```python
from build123d import *

# Parameters (mm, degrees)
F0_W     = 93.756211
F0_H     = 57.899028
F1_DEPTH = 25.4
F2_W     = 93.756211
F2_H     = 57.899028
F3_DEPTH = 7.105513
F6_DEPTH = 25.4


with BuildPart() as f1:
    # F0 (on Top) → F1 (new body)
    with BuildSketch(Plane.XY):
        with Locations((11.77345, 3.361836)):
            Rectangle(F0_W, F0_H)
        with BuildLine():
            Line((39.601556, -12.887678), (-16.054655, -12.887678))
            ThreePointArc((-16.054655, -12.887678), (-20.544783, -11.027806), (-22.404655, -6.537678))
            Line((-22.404655, -6.537678), (-22.404655, 13.26135))
            ThreePointArc((-22.404655, 13.26135), (-20.544783, 17.751478), (-16.054655, 19.61135))
            Line((-16.054655, 19.61135), (39.601556, 19.61135))
            ThreePointArc((39.601556, 19.61135), (44.091684, 17.751478), (45.951556, 13.26135))
            Line((45.951556, 13.26135), (45.951556, -6.537678))
            ThreePointArc((45.951556, -6.537678), (44.091684, -11.027806), (39.601556, -12.887678))
        make_face(mode=Mode.SUBTRACT)
    extrude(amount=F1_DEPTH)

    # F2 (on face) → F3 (join)
    with BuildSketch(Plane(origin=(0, 0, 0), x_dir=(1, 0, 0), z_dir=(0, 0, -1))):
        with Locations((11.77345, -3.361836)):
            Rectangle(F2_W, F2_H)
    extrude(amount=F3_DEPTH)

    # F5 (on face) → F6 (join)
    with BuildSketch(Plane.XY):
        with BuildLine():
            Line((-16.054655, 6.91135), (-16.054655, -0.187678))
            ThreePointArc((-16.054655, -0.187678), (-14.194783, -4.677806), (-9.704655, -6.537678))
            Line((-9.704655, -6.537678), (33.251556, -6.537678))
            ThreePointArc((33.251556, -6.537678), (37.741684, -4.677806), (39.601556, -0.187678))
            Line((39.601556, -0.187678), (39.601556, 6.91135))
            ThreePointArc((39.601556, 6.91135), (37.741684, 11.401478), (33.251556, 13.26135))
            Line((33.251556, 13.26135), (-9.704655, 13.26135))
            ThreePointArc((-9.704655, 13.26135), (-14.194783, 11.401478), (-16.054655, 6.91135))
        make_face()
    extrude(amount=F6_DEPTH)


solid = f1.part
```
Work out the finished part from the listing and answer in its coordinate system (mm). A direction names the side the tool comes from. Give positions to 0.01 mm unless a question says otherwise; leave off trailing zeros. Loops run counter-clockwise (first coordinate to the right, second up) from the corner with the lowest first, then second, coordinate; pieces in that order, holes last. Notation, with made-up numbers: (-16, 14) -> (13, 14) arc R27 ccw to (13, 35) -> close; hole circle Ø10 at (24.5, 74). An arc over 180 degrees is marked (long way). Put each result on its own line as item: value. Start each with the question number.
Item 1: The part is cut by section C-C (y = 5). Give the vertices of the cut face in (x, z).
Item 2: Which of the six approach directions +Z, -Z, +X, -X, +Y, -Y give full straight-line access (tool end or side, diameter ignored) to faces 1 (the face through (11, 23, 25.4)), 2 (the face through (-22.405, 3, 13))?
Item 3: The part is cut by section D-D (x = 42.5). Give the vertices of the cut face in (y, z).
Item 4: The mould has two halves that part along X. Classify faces 3 (the face through (44.14, -10.98, 12.52)), 4 (the face through (-35.105, 4, 9)), 5 (the face through (58.652, 4, 9)): released by +X, released by -X, zero draft, split by the parting line, or undercut.
Item 5: The part is cut by section B-B (x = 27). Give the vertices of the cut face in (y, z).
Item 6: Find the intervals of material crossed by L1, parallel to Y at x = 16, z = 3; L2, parallel to X at y = 8, z = 9; L3, parallel to X at y = 1, z = 21, in increasing order. Write a range as [from, to].
Item 7: The part is cut by section A-A (z = 22.5). Give the vertices of the cut face in (x, y).
Answers below:
1. outline: (-35.1, -7.11) -> (58.65, -7.11) -> (58.65, 25.4) -> (45.95, 25.4) -> (45.95, 0) -> (39.6, 0) -> (39.6, 25.4) -> (-16.05, 25.4) -> (-16.05, 0) -> (-22.4, 0) -> (-22.4, 25.4) -> (-35.1, 25.4) -> close
2. face 1: +Z, +X, -X, +Y, -Y
2. face 2: +Z
3. outline: (-25.59, -7.11) -> (32.31, -7.11) -> (32.31, 25.4) -> (18.91, 25.4) -> (18.91, 0) -> (-12.19, 0) -> (-12.19, 25.4) -> (-25.59, 25.4) -> close
4. face 3: undercut
4. face 4: released by -X
4. face 5: released by +X
5. outline: (-25.59, -7.11) -> (32.31, -7.11) -> (32.31, 25.4) -> (19.61, 25.4) -> (19.61, 0) -> (13.26, 0) -> (13.26, 25.4) -> (-6.54, 25.4) -> (-6.54, 0) -> (-12.89, 0) -> (-12.89, 25.4) -> (-25.59, 25.4) -> close
6. L1: [-25.59, -12.89], [-6.54, 13.26], [19.61, 32.31]
6. L2: [-35.1, -22.4], [-15.96, 39.51], [45.95, 58.65]
6. L3: [-35.1, -22.4], [-16.05, 39.6], [45.95, 58.65]
7. outline: (-35.1, -25.59) -> (58.65, -25.59) -> (58.65, 32.31) -> (-35.1, 32.31) -> close; (-16.05, -0.19) arc R6.35 ccw to (-9.7, -6.54) -> (33.25, -6.54) arc R6.35 ccw to (39.6, -0.19) -> (39.6, 6.91) arc R6.35 ccw to (33.25, 13.26) -> (-9.7, 13.26) arc R6.35 ccw to (-16.05, 6.91) -> close; hole (-22.4, -6.54) arc R6.35 ccw to (-16.05, -12.89) -> (39.6, -12.89) arc R6.35 ccw to (45.95, -6.54) -> (45.95, 13.26) arc R6.35 ccw to (39.6, 19.61) -> (-16.05, 19.61) arc R6.35 ccw to (-22.4, 13.26) -> close
